Autodesk Inventor part; units mm, degrees
ref_plane "YZ Plane" through (0, 0, 0) normal (1, 0, 0) x (0, 1, 0)
ref_plane "XZ Plane" through (0, 0, 0) normal (0, 1, 0) x (-1, 0, 0)
ref_plane "XY Plane" through (0, 0, 0) normal (0, 0, 1) x (1, 0, 0)
ref_plane "Work Plane1" through (0, 0, 0) normal (0, 0, 1) x (1, 0, 0)
sketch "Sketch1" plane through (0, 0, 0) normal (0, 0, 1) x (1, 0, 0)
  line L0 (0, 72) -> (12, 72)
  line L1 (12, 108) -> (12, 72)
  line L2 (12, 152) -> (12, 108)
  line L3 (0, 152) -> (12, 152)
  line L4 (0, 108) -> (0, 152)
  line L5 (12, 108) -> (0, 108)
  line L6 (0, 72) -> (0, 108)
  line L7 (0, 36) -> (0, 72)
  line L8 (12, 36) -> (0, 36)
  line L9 (12, 36) -> (12, 0)
  line L10 (0, 0) -> (12, 0)
  line L11 (0, -36) -> (0, 0)
  line L12 (12, -36) -> (0, -36)
  line L13 (12, 0) -> (12, -36)
  line L14 (12, 72) -> (12, 36)
  line L15 (0, 0) -> (0, 36)
  line L16 (636, -36) -> (636, -48)
  line L17 (636, -48) -> (588, -48)
  line L18 (588, -48) -> (588, -36)
  line L19 (552, -36) -> (588, -36)
  line L20 (552, -36) -> (552, -48)
  line L21 (552, -48) -> (516, -48)
  line L22 (516, -48) -> (516, -36)
  line L23 (480, -36) -> (516, -36)
  line L24 (480, -36) -> (480, -48)
  line L25 (480, -48) -> (444, -48)
  line L26 (444, -48) -> (444, -36)
  line L27 (408, -36) -> (444, -36)
  line L28 (408, -36) -> (408, -48)
  line L29 (408, -48) -> (372, -48)
  line L30 (372, -48) -> (372, -36)
  line L31 (336, -36) -> (372, -36)
  line L32 (336, -36) -> (336, -48)
  line L33 (336, -48) -> (300, -48)
  line L34 (300, -48) -> (300, -36)
  line L35 (264, -36) -> (300, -36)
  line L36 (264, -36) -> (264, -48)
  line L37 (264, -48) -> (228, -48)
  line L38 (228, -48) -> (228, -36)
  line L39 (192, -36) -> (228, -36)
  line L40 (192, -36) -> (192, -48)
  line L41 (192, -48) -> (156, -48)
  line L42 (156, -48) -> (156, -36)
  line L43 (120, -36) -> (156, -36)
  line L44 (120, -36) -> (120, -48)
  line L45 (120, -48) -> (84, -48)
  line L46 (84, -48) -> (84, -36)
  line L47 (48, -36) -> (84, -36)
  line L48 (48, -36) -> (48, -48)
  line L49 (48, -48) -> (0, -48)
  line L50 (0, -48) -> (0, -36)
  line L51 (0, -36) -> (48, -36)
  line L52 (588, -36) -> (636, -36)
  line L53 (588, -48) -> (552, -48)
  line L54 (516, -36) -> (552, -36)
  line L55 (516, -48) -> (480, -48)
  line L56 (444, -36) -> (480, -36)
  line L57 (444, -48) -> (408, -48)
  line L58 (372, -36) -> (408, -36)
  line L59 (372, -48) -> (336, -48)
  line L60 (300, -36) -> (336, -36)
  line L61 (300, -48) -> (264, -48)
  line L62 (228, -36) -> (264, -36)
  line L63 (228, -48) -> (192, -48)
  line L64 (156, -36) -> (192, -36)
  line L65 (156, -48) -> (120, -48)
  line L66 (84, -36) -> (120, -36)
  line L67 (84, -48) -> (48, -48)
  line L68 (12, 152) -> (624, 152)
  line L69 (636, -36) -> (12, -36)
  line L70 (12, -36) -> (12, 152)
  line L71 (318, 152) -> (318, 58) construction
  line L72 (318, 58) -> (636, 58) construction
  line L73 (12, 152) -> (0, 152)
  line L74 (636, 152) -> (636, 164)
  line L75 (636, 164) -> (588, 164)
  line L76 (588, 164) -> (588, 152)
  line L77 (552, 152) -> (588, 152)
  line L78 (552, 152) -> (552, 164)
  line L79 (552, 164) -> (516, 164)
  line L80 (516, 164) -> (516, 152)
  line L81 (480, 152) -> (516, 152)
  line L82 (480, 152) -> (480, 164)
  line L83 (480, 164) -> (444, 164)
  line L84 (444, 164) -> (444, 152)
  line L85 (408, 152) -> (444, 152)
  line L86 (408, 152) -> (408, 164)
  line L87 (408, 164) -> (372, 164)
  line L88 (372, 164) -> (372, 152)
  line L89 (336, 152) -> (372, 152)
  line L90 (336, 152) -> (336, 164)
  line L91 (336, 164) -> (300, 164)
  line L92 (300, 164) -> (300, 152)
  line L93 (264, 152) -> (300, 152)
  line L94 (264, 152) -> (264, 164)
  line L95 (264, 164) -> (228, 164)
  line L96 (228, 164) -> (228, 152)
  line L97 (192, 152) -> (228, 152)
  line L98 (192, 152) -> (192, 164)
  line L99 (192, 164) -> (156, 164)
  line L100 (156, 164) -> (156, 152)
  line L101 (120, 152) -> (156, 152)
  line L102 (120, 152) -> (120, 164)
  line L103 (120, 164) -> (84, 164)
  line L104 (84, 164) -> (84, 152)
  line L105 (48, 152) -> (84, 152)
  line L106 (48, 152) -> (48, 164)
  line L107 (48, 164) -> (0, 164)
  line L108 (0, 164) -> (0, 152)
  line L109 (0, 152) -> (48, 152)
  line L110 (588, 152) -> (636, 152)
  line L111 (588, 164) -> (552, 164)
  line L112 (516, 152) -> (552, 152)
  line L113 (516, 164) -> (480, 164)
  line L114 (444, 152) -> (480, 152)
  line L115 (444, 164) -> (408, 164)
  line L116 (372, 152) -> (408, 152)
  line L117 (372, 164) -> (336, 164)
  line L118 (300, 152) -> (336, 152)
  line L119 (300, 164) -> (264, 164)
  line L120 (228, 152) -> (264, 152)
  line L121 (228, 164) -> (192, 164)
  line L122 (156, 152) -> (192, 152)
  line L123 (156, 164) -> (120, 164)
  line L124 (84, 152) -> (120, 152)
  line L125 (84, 164) -> (48, 164)
  line L126 (636, 152) -> (12, 152)
  line L127 (318, 152) -> (318, -36) construction
  line L128 (636, 72) -> (624, 72)
  line L129 (624, 108) -> (624, 72)
  line L130 (624, 152) -> (624, 108)
  line L131 (636, 152) -> (624, 152)
  line L132 (636, 108) -> (636, 152)
  line L133 (624, 108) -> (636, 108)
  line L134 (636, 72) -> (636, 108)
  line L135 (636, 36) -> (636, 72)
  line L136 (624, 36) -> (636, 36)
  line L137 (624, 36) -> (624, 0)
  line L138 (636, 0) -> (624, 0)
  line L139 (636, -36) -> (636, 0)
  line L140 (624, -36) -> (636, -36)
  line L141 (624, 0) -> (624, -36)
  line L142 (624, 72) -> (624, 36)
  line L143 (636, 0) -> (636, 36)
  line L144 (636, -48) -> (636, -36)
  line L145 (624, -36) -> (624, 152)
  line L146 (624, 152) -> (636, 152)
  line L147 (636, 164) -> (636, 152)
extrude "Extrusion1" add sketch "Sketch1" along normal blind 12 contours L6 L5 L1 L0 | L1 L2 L68 L130 L129 L142 L137 L141 L52 L19 L54 L23 L56 L27 L58 L31 L60 L35 L62 L39 L64 L43 L66 L47 L51 L13 L9 L14 | L8 L9 L10 L15 | L47 L46 L67 L48 | L43 L42 L65 L44 | L35 L34 L61 L36 | L31 L30 L59 L32 | L23 L22 L55 L24 | L19 L18 L53 L20 | L133 L134 L128 L129 | L137 L136 L143 L138
ref_plane "Work Plane2" through (0, -113.0256, -190.9643) normal (-1, 0, 0) x (0, -0.5, 0.866)
ref_plane "Work Plane3" through (0, -113.0256, -190.9643) normal (-1, 0, 0) x (0, -0.5, 0.866)
sketch "Sketch3" plane through (0, 0, 12) normal (0, 0, 1) x (1, 0, 0)
  line L0 (48, -36) -> (48, -48)
  line L1 (48, -48) -> (84, -48)
  line L2 (84, -48) -> (84, -36)
  line L3 (84, -36) -> (120, -36)
  line L4 (120, -36) -> (120, -48)
  line L5 (120, -48) -> (156, -48)
  line L6 (156, -48) -> (156, -36)
  line L7 (156, -36) -> (264, -36)
  line L8 (264, -36) -> (264, -48)
  line L9 (264, -48) -> (300, -48)
  line L10 (300, -48) -> (300, -36)
  line L11 (300, -36) -> (336, -36)
  line L12 (336, -36) -> (336, -48)
  line L13 (336, -48) -> (372, -48)
  line L14 (372, -48) -> (372, -36)
  line L15 (372, -36) -> (480, -36)
  line L16 (480, -36) -> (480, -48)
  line L17 (480, -48) -> (516, -48)
  line L18 (516, -48) -> (516, -36)
  line L19 (516, -36) -> (552, -36)
  line L20 (552, -36) -> (552, -48)
  line L21 (552, -48) -> (588, -48)
  line L22 (588, -48) -> (588, -36)
  line L23 (588, -36) -> (624, -36)
  line L24 (624, -36) -> (624, 0)
  line L25 (624, 0) -> (636, 0)
  line L26 (636, 0) -> (636, 36)
  line L27 (636, 36) -> (624, 36)
  line L28 (624, 36) -> (624, 72)
  line L29 (624, 72) -> (636, 72)
  line L30 (636, 72) -> (636, 108)
  line L31 (636, 108) -> (624, 108)
  line L32 (624, 108) -> (624, 152)
  line L33 (624, 152) -> (12, 152)
  line L34 (12, 152) -> (12, 108)
  line L35 (12, 108) -> (0, 108)
  line L36 (0, 108) -> (0, 72)
  line L37 (0, 72) -> (12, 72)
  line L38 (12, 72) -> (12, 36)
  line L39 (12, 36) -> (0, 36)
  line L40 (0, 36) -> (0, 0)
  line L41 (0, 0) -> (12, 0)
  line L42 (12, 0) -> (12, -36)
  line L43 (12, -36) -> (48, -36)
properties part number "wooden_back"
CAD build for the part. Positions are in the model's coordinates, mm. A direction names the side the tool comes from. Round coordinates to 2 decimals unless told otherwise and drop trailing zeros. Write each loop counter-clockwise with the first axis right and the second up, starting at its lowest first coordinate (ties: lowest second). Pieces come first, ordered by that corner, then holes. Notation, with made-up numbers: (47, 71) -> (60, 71) arc R31 ccw to (60, 104) -> close; hole circle Ø6 at (81, -29). An arc over 180 degrees is marked (long way). Answer as a JSON object with one key per item and string values.
(1) Probe probe 1 along X at (y, z) = (42.5, 7.5); probe 2 along Y at (x, z) = (520, 5). List the from-to ranges inside material, lowest first. Write a range as [from, to].
Reported:
{"probe 1": "x = [12, 624]", "probe 2": "y = [-36, 152]"}
(2) Which spindle directions (+Z, -Z, +X, -X, +Y, -Y) get a long thin tool onto all of the face, cutting with end or side? Do faces 4 (the face through (12, 130, 6)), 5 (the face through (6, 0, 6)), 6 (the face through (624, 130, 6)), 7 (the face through (624, -18, 6)), 8 (the face through (300, -42, 6)). Say none if no direction does.
Reported:
{"face 4": "+Z, -Z, -X, +Y", "face 5": "+Z, -Z, -X, -Y", "face 6": "+Z, -Z, +X, +Y", "face 7": "+Z, -Z, +X, -Y", "face 8": "+Z, -Z, -Y"}
(3) Pin check, flat tips, straight feed: P1, Ø6, axis at y = 46.5, z = 4.5, coming from the +X side; P2, Ø3.5, axis at y = -41.5, z = 4, coming from the -X side; P3, Ø3.5, axis at x = 5.5, z = 5.5, coming from the -Y side. Stop position of each tip, or through.
Reported:
{"P1": "stops at x = 624", "P2": "stops at x = 48", "P3": "stops at y = 0"}
(4) Band-saw the part on A-A, the plane y = 52. List the corners of the cut face in (x, z).
Reported:
{"outline": "(12, 0) -> (624, 0) -> (624, 12) -> (12, 12) -> close"}
(5) Band-saw the part on B-B, the plane x = 219. List the corners of the cut face in (y, z), then the cut area to 3 significant figures.
Reported:
{"outline": "(-36, 0) -> (152, 0) -> (152, 12) -> (-36, 12) -> close", "area": "2,260 mm^2"}
(6) Two-plate mould, pull along Y, no slides. Class faces 1 (the face through (156, -42, 6)), 2 (the face through (606, -36, 6)), 3 (the face through (624, 54, 6)): +Y half, -Y half, draft (parallel to the pull), parting line (faces both ways), or undercut.
Reported:
{"face 1": "draft", "face 2": "-Y half", "face 3": "undercut"}
